from build123d import *

# Parameters (mm, degrees)
F0_W     = 38.1
F0_H     = 38.1
F0_W_2   = 28.5496
F0_H_2   = 28.5496
F1_DEPTH = 609.6
F3_DEPTH = 38.101
F4_R     = 6.35
F5_DEPTH = 38.101


with BuildPart() as f1:
    # F0 (on Right) → F1 (new body)
    with BuildSketch(Plane.YZ):
        Rectangle(F0_W, F0_H)
        Rectangle(F0_W_2, F0_H_2, mode=Mode.SUBTRACT)
    extrude(amount=F1_DEPTH)

    # F2 (on face) → F3 (cut, through all)
    with BuildSketch(Plane(origin=(0, 19.05, 0), x_dir=(-1, 0, 0), z_dir=(0, 1, 0))):
        Polygon((0, -19.05), (0, 19.05), (-38.1, -19.05), align=None)
    extrude(amount=-F3_DEPTH, mode=Mode.SUBTRACT)

    # F4 (on face) → F5 (cut, through all)
    with BuildSketch(Plane(origin=(0, 19.05, 0), x_dir=(-1, 0, 0), z_dir=(0, 1, 0))):
        with Locations((-558.8, 0)):
            Circle(F4_R)
    extrude(amount=-F5_DEPTH, mode=Mode.SUBTRACT)


solid = f1.part
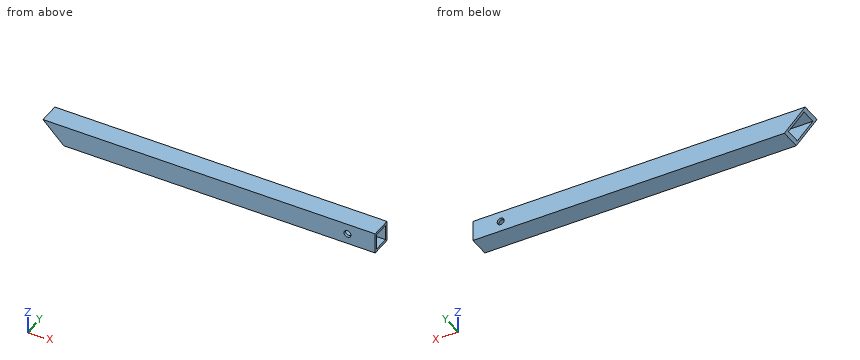
Design review of the part built by this model. Coordinates are the model's own, in mm. Coordinates: 2 decimals unless noted, no trailing zeros. Loops run counter-clockwise (first coordinate to the right, second up) from the corner with the lowest first, then second, coordinate; pieces in that order, holes last. Notation, with made-up numbers: M -9,53.5 L 27,53.5 A12 cw 27,74.5 Z; hole C 80.25,-13 d8. An arc over 180 degrees is marked long. Answer as CSV lines item,"result".
Item 1: Add section B-B on z = 0. State the section outline as (x, y) points, plus the area to 3 significant figures.
Answer list:
outline,"M 19.05,-19.05 L 552.45,-19.05 L 552.45,-14.27 L 19.05,-14.27 Z; M 19.05,14.27 L 552.45,14.27 L 552.45,19.05 L 19.05,19.05 Z; M 565.15,-19.05 L 609.6,-19.05 L 609.6,-14.27 L 565.15,-14.27 Z; M 565.15,14.27 L 609.6,14.27 L 609.6,19.05 L 565.15,19.05 Z"
area,"5,520 mm²"
Item 2: For probe 1 along Z at (x, y) = (558, 16); probe 2 along Y at (x, z) = (179.5, -11.5), list the stretches that pass through material, from the lowest coordinate up.
Answer list:
probe 1,"-19.05 to -6.3, 6.3 to 19.05"
probe 2,"-19.05 to -14.27, 14.27 to 19.05"
Item 3: Add section A-A on x = 558.8. State the section outline as (y, z) points, plus the area to 3 significant figures.
Answer list:
outline,"M -19.05,-19.05 L 19.05,-19.05 L 19.05,-6.35 L 14.27,-6.35 L 14.27,-14.27 L -14.27,-14.27 L -14.27,-6.35 L -19.05,-6.35 Z; M -19.05,6.35 L -14.27,6.35 L -14.27,14.27 L 14.27,14.27 L 14.27,6.35 L 19.05,6.35 L 19.05,19.05 L -19.05,19.05 Z"
area,"515 mm²"
Item 4: For P1, Ø11.5, axis at x = 558.8, z = 0, coming from the +Y side, flat-tipped, find the tip position at first contact; note if it passes through.
Answer list:
P1,"through"
Item 5: Add section C-C on y = 7. State the section outline as (x, z) points.
Answer list:
outline,"M 0,19.05 L 4.78,14.27 L 609.6,14.27 L 609.6,19.05 Z; M 33.32,-14.27 L 38.1,-19.05 L 609.6,-19.05 L 609.6,-14.27 Z"
Item 6: Add section D-D on x = 239.5. State the section outline as (y, z) points, plus the area to 3 significant figures.
Answer list:
outline,"M -19.05,-19.05 L 19.05,-19.05 L 19.05,19.05 L -19.05,19.05 Z; hole M -14.27,-14.27 L 14.27,-14.27 L 14.27,14.27 L -14.27,14.27 Z"
area,"637 mm²"
